Can you work these out from the model? Positions are in its coordinate system, mm. A direction names the side the tool comes from. Round coordinates to 2 decimals unless told otherwise and drop trailing zeros. Loops run counter-clockwise (first coordinate to the right, second up) from the corner with the lowest first, then second, coordinate; pieces in that order, holes last.
(1) Thinking about a two-plate mould opening in Z: for faces 3 (the face through (-2, -2, 0)), 4 (the face through (0, -7.35, 3)), 5 (the face through (-8, 0, 8)), 6 (the face through (0, 9, 4)), which applies, released by +Z, released by -Z, zero draft, split by the parting line, or undercut?
(2) If I drill on line 1 along X through (y, z) = (2.5, 3.25); line 2 along Y through (x, z) = (-2.5, 2.5); line 3 along X through (y, z) = (3, 7.75), over which ranges is the centre line in solid material (lowest first)?
(3) Will these pins go through, and if not, where does the flat tip stop? pin 1 Ø3 at (x, y) = (0, 0) entering from +Z; pin 2 Ø3 at (x, y) = (5.1, 0) entering from +Z.
(4) I want a section at D-D on y = 0. Write out the boundary of the cut face in (x, z).
(5) Which directions (+Z, -Z, +X, -X, +Y, -Y) give clear straight access to the entire face, cutting with the end or side of a thin tool? Please do faces 1 (the face through (9, 0, 4)), 2 (the face through (0, 7, 6)).
(6) I want a section at A-A on z = 1.75. Write out the boundary of the cut face in (x, y).
(7) I want a section at C-C on y = 2.25. Write out the boundary of the cut face in (x, z), plus the area to 3 significant figures.
(8) I want a section at B-B on x = -5.1. Write out the boundary of the cut face in (y, z).
from build123d import *

# Parameters (mm, degrees)
F0_W     = 14
F0_H     = 14
F0_R     = 0.9
F0_R_2   = 0.75
F0_R_3   = 2
F1_DEPTH = 2
F0_W_2   = 15.7
F0_H_2   = 15.9
F3_DEPTH = 7
F0_W_3   = 18
F0_H_3   = 18
F4_DEPTH = 8
F5_W     = 14
F5_H     = 14.7
F6_DEPTH = 2.5


with BuildPart() as f1:
    # F0 (on Top) → F1 (new body)
    with BuildSketch(Plane.XY):
        Rectangle(F0_W, F0_H)
        with Locations((-5.1, 0)):
            Circle(F0_R, mode=Mode.SUBTRACT)
        with Locations((-3.5, 2.25)):
            Circle(F0_R_2, mode=Mode.SUBTRACT)
        Circle(F0_R_3, mode=Mode.SUBTRACT)
        with Locations((5.1, 0)):
            Circle(F0_R, mode=Mode.SUBTRACT)
        with Locations((2, 5.5)):
            Circle(F0_R_2, mode=Mode.SUBTRACT)
    extrude(amount=F1_DEPTH)

    # F0 (on Top) → F3 (join)
    with BuildSketch(Plane.XY):
        Rectangle(F0_W_2, F0_H_2)
        Rectangle(F0_W, F0_H, mode=Mode.SUBTRACT)
    extrude(amount=F3_DEPTH)

    # F0 (on Top) → F4 (join)
    with BuildSketch(Plane.XY):
        Rectangle(F0_W_3, F0_H_3)
        Rectangle(F0_W_2, F0_H_2, mode=Mode.SUBTRACT)
    extrude(amount=F4_DEPTH)

    # F5 (on offset) → F6 (cut, through all)
    with BuildSketch(Plane.XY.offset(4.5)):
        Rectangle(F5_W, F5_H)
    extrude(amount=-F6_DEPTH, mode=Mode.SUBTRACT)


solid = f1.part
Filled sheet:
1. face 3: released by -Z
1. face 4: undercut
1. face 5: released by +Z
1. face 6: zero draft
2. line 1: x = -9 to -7, 7 to 9
2. line 2: y = -9 to -7.35, 7.35 to 9
2. line 3: x = -9 to -7.85, 7.85 to 9
3. pin 1: passes through
3. pin 2: stops at z = 2
4. outline: (-9, 0) - (-6, 0) - (-6, 2) - (-7, 2) - (-7, 7) - (-7.85, 7) - (-7.85, 8) - (-9, 8) - close; (-4.2, 0) - (-2, 0) - (-2, 2) - (-4.2, 2) - close; (2, 0) - (4.2, 0) - (4.2, 2) - (2, 2) - close; (6, 0) - (9, 0) - (9, 8) - (7.85, 8) - (7.85, 7) - (7, 7) - (7, 2) - (6, 2) - close
5. face 1: +Z, -Z, +X, +Y, -Y
5. face 2: +Z
6. outline: (-9, -9) - (9, -9) - (9, 9) - (-9, 9) - close; hole circle Ø1.8 at (-5.1, 0); hole circle Ø1.5 at (-3.5, 2.25); hole circle Ø4 at (0, 0); hole circle Ø1.5 at (2, 5.5); hole circle Ø1.8 at (5.1, 0)
7. outline: (-9, 0) - (-4.25, 0) - (-4.25, 2) - (-7, 2) - (-7, 7) - (-7.85, 7) - (-7.85, 8) - (-9, 8) - close; (-2.75, 0) - (9, 0) - (9, 8) - (7.85, 8) - (7.85, 7) - (7, 7) - (7, 2) - (-2.75, 2) - close
7. area: 55.3 mm2
8. outline: (-9, 0) - (-0.9, 0) - (-0.9, 2) - (-7.35, 2) - (-7.35, 4.5) - (-7, 4.5) - (-7, 7) - (-7.95, 7) - (-7.95, 8) - (-9, 8) - close; (0.9, 0) - (9, 0) - (9, 8) - (7.95, 8) - (7.95, 7) - (7, 7) - (7, 4.5) - (7.35, 4.5) - (7.35, 2) - (0.9, 2) - close
